Check sheet for the drawn part. Datum: minimum x, y, z corner. Units: mm. Coordinates: 2 decimals unless noted, no trailing zeros. Loops run counter-clockwise (first coordinate to the right, second up) from the corner with the lowest first, then second, coordinate; pieces in that order, holes last.
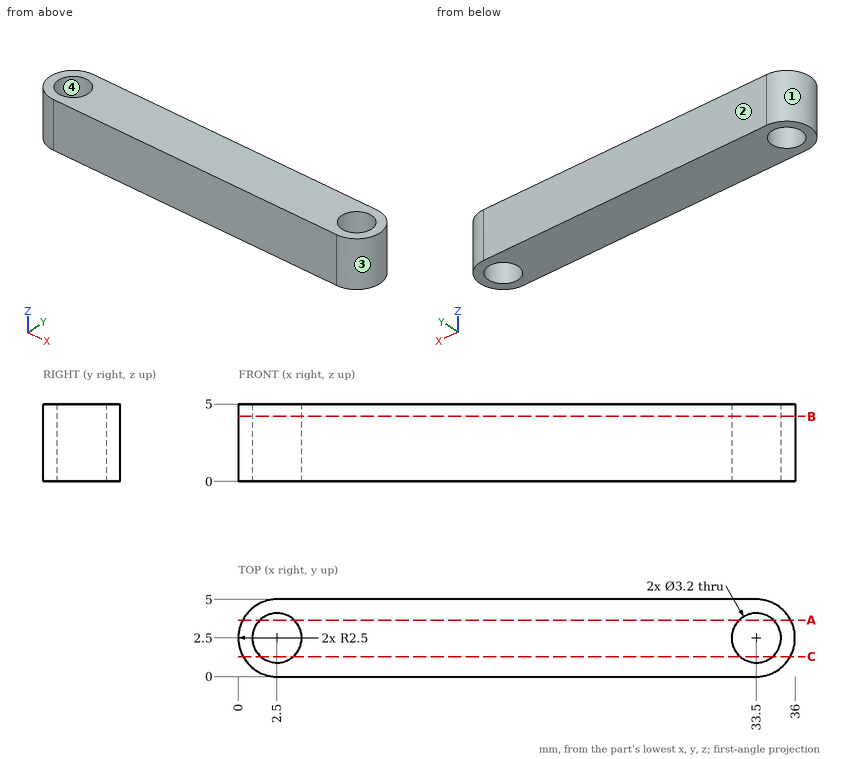
1) Section check B-B on z = 4.2. Enter the section's corners in (x, y).
Answer sheet:
outline: (2.5, 0) - (33.5, 0) arc R2.5 ccw to (33.5, 5) - (2.5, 5) arc R2.5 ccw to start; hole circle Ø3.2 at (2.5, 2.5); hole circle Ø3.2 at (33.5, 2.5)
2) Section check A-A on y = 3.65. Enter the section's corners in (x, z), plus the area to 3 significant figures.
Answer sheet:
outline: (0.28, 0) - (1.39, 0) - (1.39, 5) - (0.28, 5) - close; (3.61, 0) - (32.39, 0) - (32.39, 5) - (3.61, 5) - close; (34.61, 0) - (35.72, 0) - (35.72, 5) - (34.61, 5) - close
area: 155 mm2
3) Mould release check, pull along X, two halves, no side actions. Record for the marked faces 1, 2, 3 and 4: +X half, -X half, draft (parallel to the pull), parting line (faces both ways), or undercut.
Answer sheet:
face 1: -X half
face 2: draft
face 3: +X half
face 4: undercut
4) Scan lines: line 1 (X direction, y = 1.3, z = 0.3); line 2 (Y direction, x = 33.5, z = 3.7); line 3 (X direction, y = 3.95, z = 2.9). Record each from-to range of solid material in increasing order.
Answer sheet:
line 1: x = 0.31 to 1.44, 3.56 to 32.44, 34.56 to 35.69
line 2: y = 0 to 0.9, 4.1 to 5
line 3: x = 0.46 to 1.82, 3.18 to 32.82, 34.18 to 35.54
5) Depth check by flat-ended pin: pin 1 (2 mm diameter, centred on y = 3.5, z = 2, fed in from -X). Enter the tip coordinate at first touch or a pass-through.
Answer sheet:
pin 1: stops at x = 0
6) Section check C-C on y = 1.3. Enter the section's corners in (x, z).
Answer sheet:
outline: (0.31, 0) - (1.44, 0) - (1.44, 5) - (0.31, 5) - close; (3.56, 0) - (32.44, 0) - (32.44, 5) - (3.56, 5) - close; (34.56, 0) - (35.69, 0) - (35.69, 5) - (34.56, 5) - close
